Read the model definition and answer for the solid it produces. Units are mm, in the model's axes. A direction names the side the tool comes from. Coordinates: 2 decimals unless noted, no trailing zeros. Loops run counter-clockwise (first coordinate to the right, second up) from the corner with the lowest first, then second, coordinate; pieces in that order, holes last. Notation, with made-up numbers: M 17.25,-12 L 28.25,-12 A5 ccw 28.25,-3 Z; hole C 1,86.5 d7. An arc over 180 degrees is marked long. Put each result on its own line as item: value.
from build123d import *

# Parameters (mm, degrees)
SKETCH1_W           = 124.5
SKETCH1_H           = 78.9
BOSS_EXTRUDE1_DEPTH = 1
SKETCH2_R           = 3.5
BOSS_EXTRUDE2_DEPTH = 4
SKETCH3_R           = 1.75
BOSS_EXTRUDE3_DEPTH = 3


with BuildPart() as part:
    # Sketch1 → Boss-Extrude1 (new body)
    with BuildSketch(Plane.XY):
        with Locations((-15, -5.25)):
            Rectangle(SKETCH1_W, SKETCH1_H)
    extrude(amount=BOSS_EXTRUDE1_DEPTH)

    # Sketch2 → Boss-Extrude2 (add)
    with BuildSketch(Plane.XY.offset(1)):
        with Locations(Location((-68.25, 27.75, 0), (0, 0, 180))):
            Circle(SKETCH2_R)
        with Locations(Location((23.75, 27.75, 0), (0, 0, 180))):
            Circle(SKETCH2_R)
        with Locations(Location((23.75, -38.25, 0), (0, 0, 180))):
            Circle(SKETCH2_R)
        with Locations(Location((-68.25, -38.25, 0), (0, 0, 180))):
            Circle(SKETCH2_R)
    extrude(amount=BOSS_EXTRUDE2_DEPTH)

    # Sketch3 → Boss-Extrude3 (add)
    with BuildSketch(Plane.XY.offset(5)):
        with Locations((-68.25, 27.75)):
            Circle(SKETCH3_R)
        with Locations((23.75, 27.75)):
            Circle(SKETCH3_R)
        with Locations((23.75, -38.25)):
            Circle(SKETCH3_R)
        with Locations((-68.25, -38.25)):
            Circle(SKETCH3_R)
    extrude(amount=BOSS_EXTRUDE3_DEPTH)


solid = part.part
1) Find section C-C, the plane z = 6.5. Write down the section's boundary in (x, y).
Answer list:
outline: C -68.25,-38.25 d3.5; C -68.25,27.75 d3.5; C 23.75,-38.25 d3.5; C 23.75,27.75 d3.5
2) Find section A-A, the plane x = 23.75. Write down the section's boundary in (y, z), plus the area to 3 significant figures.
Answer list:
outline: M -44.7,0 L 34.2,0 L 34.2,1 L 31.25,1 L 31.25,5 L 29.5,5 L 29.5,8 L 26,8 L 26,5 L 24.25,5 L 24.25,1 L -34.75,1 L -34.75,5 L -36.5,5 L -36.5,8 L -40,8 L -40,5 L -41.75,5 L -41.75,1 L -44.7,1 Z
area: 156 mm^2
3) Find section B-B, the plane y = 27.75. Write down the section's boundary in (x, z).
Answer list:
outline: M -77.25,0 L 47.25,0 L 47.25,1 L 27.25,1 L 27.25,5 L 25.5,5 L 25.5,8 L 22,8 L 22,5 L 20.25,5 L 20.25,1 L -64.75,1 L -64.75,5 L -66.5,5 L -66.5,8 L -70,8 L -70,5 L -71.75,5 L -71.75,1 L -77.25,1 Z
4) Given pin 1 Ø1 at (x, y) = (-43.5, 12) entering from +Z, flat-ended and moving along its own axis, determine where the tip first touches the part or whether it passes through.
Answer list:
pin 1: stops at z = 1
5) Determine the mould class of faces 1 (the flat face through (-16, -5, 0)), 2 (the cylindrical face through (22.36, -39.31, 6.48)) for opening direction X: released by +X, released by -X, zero draft, split by the parting line, or undercut.
Answer list:
face 1: zero draft
face 2: undercut
6) Straight lines are drawn through the part: line 1 (Z direction, x = 17.5, y = 17); line 2 (X direction, y = 28, z = 4.75); line 3 (Y direction, x = -68, z = 5.25). For each, find the intervals that lie inside material, in ascending order. Write a range as [from, to].
Answer list:
line 1: z = [0, 1]
line 2: x = [-71.74, -64.76], [20.26, 27.24]
line 3: y = [-39.98, -36.52], [26.02, 29.48]
7) Which of the six approach directions +Z, -Z, +X, -X, +Y, -Y give full straight-line access (tool end or side, diameter ignored) to faces 3 (the flat face through (-68, -38, 8)), 4 (the flat face through (-69, -40, 5))?
Answer list:
face 3: +Z, +X, -X, +Y, -Y
face 4: +Z
8) Find section D-D, the plane y = -16.5. Write down the section's boundary in (x, z).
Answer list:
outline: M -77.25,0 L 47.25,0 L 47.25,1 L -77.25,1 Z
